```python
from build123d import *

# Parameters (mm, degrees)
BOSS_EXTRUDE1_DEPTH = 19.05
SKETCH4_W           = 19.05
SKETCH4_H           = 50.8
BOSS_EXTRUDE2_DEPTH = 19.05
FILLET1_R           = 2.54
SKETCH2_R           = 3.175
CUT_EXTRUDE1_DEPTH  = 186.893470837
FILLET2_R           = 25.4
FILLET3_R           = 25.4
FILLET4_R           = 6.35
FILLET5_R           = 9.525
SKETCH6_R           = 2.286
CUT_EXTRUDE3_DEPTH  = 186.893470837
CHAMFER1_SIZE       = 3.175


with BuildPart() as part:
    # Sketch1 → Boss-Extrude1 (new body)
    with BuildSketch(Plane.XY):
        Polygon((0, 0), (177.8, 0), (177.8, 44.45), (33.749441782, 19.05), (0, 19.05), align=None)
    extrude(amount=BOSS_EXTRUDE1_DEPTH)

    # Sketch4 → Boss-Extrude2 (add)
    with BuildSketch(Plane.XY.offset(19.05)):
        with Locations((9.525, -25.4)):
            Rectangle(SKETCH4_W, SKETCH4_H)
    extrude(amount=-BOSS_EXTRUDE2_DEPTH)

    # Fillet1
    fillet1_edges = [part.edges().sort_by_distance(p)[0] for p in [
        (33.749441782, 19.05, 9.525),
        (177.8, 44.45, 9.525),
    ]]
    fillet(fillet1_edges, radius=FILLET1_R)

    # Sketch2 → Cut-Extrude1 (cut, through all)
    with BuildSketch(Plane.XY.offset(19.05)):
        with Locations((9.525, -41.275)):
            Circle(SKETCH2_R)
    extrude(amount=-CUT_EXTRUDE1_DEPTH, mode=Mode.SUBTRACT)

    # Fillet2
    fillet2_edges = [part.edges().sort_by_distance(p)[0] for p in [
        (177.8, 0, 9.525),
    ]]
    fillet(fillet2_edges, radius=FILLET2_R)

    # Fillet3
    fillet3_edges = [part.edges().sort_by_distance(p)[0] for p in [
        (0, 19.05, 9.525),
    ]]
    fillet(fillet3_edges, radius=FILLET3_R)

    # Fillet4
    fillet4_edges = [part.edges().sort_by_distance(p)[0] for p in [
        (19.05, 0, 9.525),
    ]]
    fillet(fillet4_edges, radius=FILLET4_R)

    # Fillet5
    fillet5_edges = [part.edges().sort_by_distance(p)[0] for p in [
        (19.05, -50.8, 9.525),
        (0, -50.8, 9.525),
    ]]
    fillet(fillet5_edges, radius=FILLET5_R - 0.0001)  # a hair under: the kernel refuses the full size

    # Sketch6 → Cut-Extrude3 (cut, through all)
    with BuildSketch(Plane.XY.offset(19.05)):
        with Locations((13.952511732, 9.331690663)):
            Circle(SKETCH6_R)
    extrude(amount=-CUT_EXTRUDE3_DEPTH, mode=Mode.SUBTRACT)

    # Chamfer1
    chamfer1_edges = [part.edges().sort_by_distance(p)[0] for p in [
        (11.666511732, 9.331690663, 19.05),
    ]]
    chamfer(chamfer1_edges, length=CHAMFER1_SIZE)


solid = part.part
```
The model under review builds one solid part; all positions refer to its coordinate system, in mm. A direction names the side the tool comes from. Round coordinates to 2 decimals unless told otherwise and drop trailing zeros. Loops run counter-clockwise (first coordinate to the right, second up) from the corner with the lowest first, then second, coordinate; pieces in that order, holes last.
Item 1: Take a section at A-A (y = -33.5). Write out the cut boundary in (x, z).
Determined:
outline: (0, 0) - (19.05, 0) - (19.05, 19.05) - (0, 19.05) - close
Item 2: Clearance check with flat-ended pins moving along their axes: pin 1 Ø3.5 at (x, y) = (13.95, 9.33) entering from +Z; pin 2 Ø6.5 at (x, z) = (30, 6) entering from +Y; pin 3 Ø3 at (x, z) = (133, 12) entering from -Y; pin 4 Ø8 at (x, z) = (154.5, 15) entering from +Y. State where each tip first meets the part, or that it passes through.
Determined:
pin 1: passes through
pin 2: stops at y = 19.05
pin 3: stops at y = 0
pin 4: stops at y = 41.05
Item 3: For faces 1 (the face through (11.67, 9.43, 8.05)), 2 (the face through (88, 0, 9)), 3 (the face through (30, 19.05, 9)), list the 3-axis set-ups (+Z, -Z, +X, -X, +Y, -Y) from which the entire face can be reached by the end or side of a thin tool; tool diameter is ignored.
Determined:
face 1: +Z, -Z
face 2: +Z, -Z, +X, -Y
face 3: +Z, -Z, -X, +Y
Item 4: Mouldability with a two-part tool opening along Y and no side actions: class faces 4 (the face through (2.86, -48.08, 9.39)), 5 (the face through (16.28, 10.06, 16.03)), 6 (the face through (177.8, 33, 9)) as released by +Y, released by -Y, zero draft, split by the parting line, or undercut.
Determined:
face 4: released by -Y
face 5: undercut
face 6: zero draft
Item 5: For line 1 (Y direction, x = 8, z = 2); line 2 (X direction, y = -34, z = 3.75), list the stretches that pass through material, from the lowest coordinate up.
Determined:
line 1: y = -50.68 to -44.06, -38.49 to 12.15
line 2: x = 0 to 19.05
Item 6: Take a section at C-C (x = 107.5). Write out the cut boundary in (y, z).
Determined:
outline: (0, 0) - (32.05, 0) - (32.05, 19.05) - (0, 19.05) - close
Item 7: Take a section at B-B (z = 9.75). Give the number of separate pieces and of enclosed holes in the cut face, then the cut area to 3 significant figures.
Determined:
separate pieces: 1
enclosed holes: 2
area: 5,830 mm2
